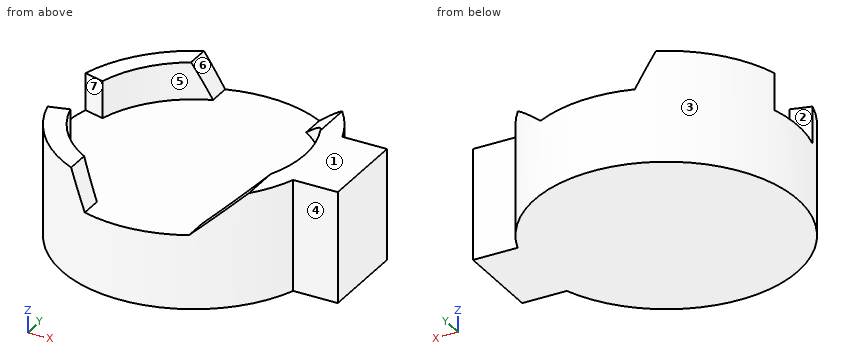
```python
from build123d import *

# Parameters (mm, degrees)
PAD063_DEPTH    = 9
SKETCH096_R     = 9
POCKET019_DEPTH = 3
POCKET020_DEPTH = 24.2527662109
POCKET021_DEPTH = 3


with BuildPart() as part:
    # Sketch095 → Pad063 (new body)
    with BuildSketch(Plane.XY.offset(1.6)):
        with BuildLine():
            Line((64.6986240714, 66.789096024), (68.3068088834, 66.789096024))
            Line((68.3068088834, 66.789096024), (68.3068088834, 59.6371823367))
            Line((68.3068088834, 59.6371823367), (64.6946039998, 59.6371823367))
            ThreePointArc((64.6986240714, 66.789096024), (43.973359138, 63.2247876667), (64.6946039998, 59.6371823367))
        make_face()
    extrude(amount=PAD063_DEPTH)

    # Sketch096 (on Face6 of Pad063) → Pocket019 (cut)
    with BuildSketch(Plane.XY.offset(10.6)):
        with Locations((54.643516, 63.21879)):
            Circle(SKETCH096_R)
    extrude(amount=-POCKET019_DEPTH, mode=Mode.SUBTRACT)

    # Sketch097 (on DatumPlane) → Pocket020 (cut, through all)
    with BuildSketch(Plane(origin=(0, 49.6371823367, 1.6), x_dir=(1, 0, 0), z_dir=(0, -1, 0))):
        Polygon((47.624802, 14.26), (51.504802, 6), (59.534802, 6), (66.034802, 11.82), align=None)
    extrude(amount=-POCKET020_DEPTH, mode=Mode.SUBTRACT)

    # Sketch098 (on Face10 of Pocket020) → Pocket021 (cut)
    with BuildSketch(Plane.XY.offset(10.6)):
        Polygon((54.643516, 63.21879), (36.6761624803, 68.0350836562), (36.6761624803, 58.4024963438), align=None)
    extrude(amount=-POCKET021_DEPTH, mode=Mode.SUBTRACT)


with BuildPart() as part_1:
    # Body011 placement: moved
    add(part.part.moved(Location((0, 0, 20))))


solid = part_1.part
```
Input: part model. Units: mm. Frame: model coordinates. Face numbers are marked on the shaded views. A direction names the side the tool comes from. Round coordinates to 2 decimals unless told otherwise and drop trailing zeros. Loops run counter-clockwise (first coordinate to the right, second up) from the corner with the lowest first, then second, coordinate; pieces in that order, holes last. Notation, with made-up numbers: (-22, -36) - (23, -36) arc R16 cw to (23, -28) - close; hole circle Ø9 at (83.5, 53). An arc over 180 degrees is marked (long way). One line per item, written item: value. Start each with the question number.
(1) Contact query for flat-ended pins moving along their axis: P1, Ø4, axis at x = 66.5, z = 27.5, coming from the -Y side; P2, Ø1, axis at x = 53.5, z = 25.5, coming from the +Y side; P3, Ø2, axis at x = 52.5, z = 25, coming from the -Y side. Output: stop coordinate, or through.
(2) Access query for the marked faces 4, 5, 6 and 7. Directions: +Z, -Z, +X, -X, +Y, -Y. A direction counts if a zero-diameter tool reaches every point of the face in a straight line with its end or side. Return the directions, or none.
(3) Draft query along Y for the marked faces 1, 2 and 3. Return one class per face: +Y half, -Y half, draft (parallel to the pull), parting line (faces both ways), or undercut.
(4) Section A-A, the plane z = 29. Return loops of the section in (x, y), plus the area to 3 significant figures.
(5) Ray query, line 1 (Z direction, x = 59, y = 63); line 2 (X direction, y = 69, z = 28.25); line 3 (Y direction, x = 51.25, z = 27.75). Return the intervals inside material, ascending. Write a range as [from, to].
(6) Section C-C, the plane x = 46.75. Return loops of the section in (y, z).
(7) Section B-B, the plane y = 59. Return loops of the section in (x, z), plus the area to 3 significant figures.
(8) Section D-D, the plane z = 23. Return loops of the section in (x, y), plus the area to 3 significant figures.
Results below:
1. P1: y = 59.13
1. P2: y = 73.87
1. P3: y = 52.61
2. face 4: +Z, -Z, +X, -Y
2. face 5: +Z
2. face 6: +Z, +Y, -Y
2. face 7: +Z, -X
3. face 1: draft
3. face 2: undercut
3. face 3: parting line
4. outline: (44.34, 60.46) arc R10.67 ccw to (50.85, 53.25) - (50.85, 55.06) arc R9 cw to (45.95, 60.89) - close; (44.34, 65.98) - (45.95, 65.55) arc R9 cw to (50.85, 71.38) - (50.85, 73.19) arc R10.67 ccw to start; (61.1, 54.72) arc R10.67 ccw to (64.69, 59.64) - (68.31, 59.64) - (68.31, 66.79) - (64.7, 66.79) arc R10.67 ccw to (61.1, 71.72) - (61.1, 69.49) arc R9 cw to (61.1, 56.95) - close
4. area: 80.9 mm^2
5. line 1: [21.6, 27.6]
5. line 2: [45.68, 47.75], [61.54, 63.61]
5. line 3: [53.1, 54.88], [71.55, 73.33]
6. outline: (56.04, 21.6) - (70.4, 21.6) - (70.4, 30.6) - (67.54, 30.6) - (67.54, 27.6) - (58.9, 27.6) - (58.9, 30.6) - (56.04, 30.6) - close
7. outline: (44.84, 21.6) - (64.44, 21.6) - (64.44, 30.6) - (62.89, 30.6) - (62.59, 30.34) - (62.59, 27.6) - (46.69, 27.6) - (46.69, 30.6) - (44.84, 30.6) - close
7. area: 129 mm^2
8. outline: (64.69, 59.64) - (68.31, 59.64) - (68.31, 66.79) - (64.7, 66.79) arc R10.67 ccw (long way) to start
8. area: 381 mm^2
